```python
from build123d import *

# Parameters (mm, degrees)
SKETCH1_W           = 30
SKETCH1_H           = 100
BOSS_EXTRUDE1_DEPTH = 3.75
BOSS_EXTRUDE2_START = -3
SKETCH2_W           = 15
SKETCH2_H           = 50
BOSS_EXTRUDE2_DEPTH = 4


with BuildPart() as part:
    # Sketch1 → Boss-Extrude1 (new, symmetric)
    with BuildSketch(Plane(origin=(0, 0, 0), x_dir=(1, 0, 0), z_dir=(0, 1, 0))):
        with Locations((-15, 0)):
            Rectangle(SKETCH1_W, SKETCH1_H)
    extrude(amount=BOSS_EXTRUDE1_DEPTH, both=True)

    # Sketch2 → Boss-Extrude2 (add)
    with BuildSketch(Plane(origin=(0, 3.75, 0), x_dir=(1, 0, 0), z_dir=(0, 1, 0)).offset(BOSS_EXTRUDE2_START)):
        with Locations((7.5, 0)):
            Rectangle(SKETCH2_W, SKETCH2_H)
    extrude(amount=-BOSS_EXTRUDE2_DEPTH)


solid = part.part
```
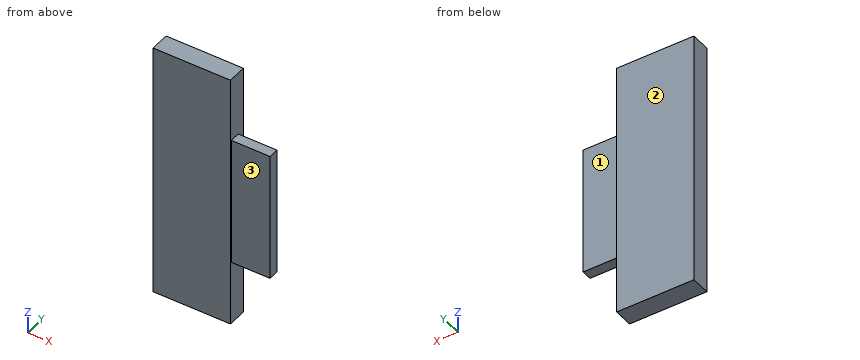
Source: CAD feature listing. Evaluate the final solid. Frame: model axes, mm. Face numbers are marked on the shaded views. A direction names the side the tool comes from. Coordinates: 2 decimals unless noted, no trailing zeros. Loops run counter-clockwise (first coordinate to the right, second up) from the corner with the lowest first, then second, coordinate; pieces in that order, holes last. Notation, with made-up numbers: M -20,17.25 L 39,17.25 A19 ccw 39,26.25 Z; hole C 57,36 d10. An arc over 180 degrees is marked long. Use CSV: the item, a comma, the result in double quotes.
(1) Cut plane C-C on x = 9. Return loops of the section in (y, z), and give its area (3 significant figures).
Answers follow:
outline,"M -3.25,-25 L 0.75,-25 L 0.75,25 L -3.25,25 Z"
area,"200 mm²"
(2) Cut plane D-D on z = 44. Return loops of the section in (x, y), and give its area (3 significant figures).
Answers follow:
outline,"M -30,-3.75 L 0,-3.75 L 0,3.75 L -30,3.75 Z"
area,"225 mm²"
(3) Line query: line 1 (X direction, y = 3, z = 31); line 2 (Z direction, x = 5, y = -0.25). Output: solid intervals per line, ascending. Write a range as [from, to].
Answers follow:
line 1,"[-30, 0]"
line 2,"[-25, 25]"
(4) Reachability of the marked faces 1, 2 and 3 from +Z, -Z, +X, -X, +Y, -Y: full face, straight path, thin tool, end or side. Return the list, or none.
Answers follow:
face 1,"+Z, -Z, +X, +Y"
face 2,"+Z, -Z, +X, -X, +Y"
face 3,"+Z, -Z, +X, -Y"
(5) Contact query for flat-ended pins moving along their axis: pin 1 (3 mm diameter, centred on x = 5.5, y = -1.5, fed in from -Z); pin 2 (3 mm diameter, centred on x = 0.5, z = -35.5, fed in from -Y); pin 3 (7.5 mm diameter, centred on x = 6.5, z = 6, fed in from +Y); pin 4 (1.2 mm diameter, centred on x = 10, y = -0.5, fed in from +Z). Output: stop coordinate, or through.
Answers follow:
pin 1,"z = -25"
pin 2,"y = -3.75"
pin 3,"y = 0.75"
pin 4,"z = 25"
(6) Cut plane B-B on z = -24. Return loops of the section in (x, y), and give its area (3 significant figures).
Answers follow:
outline,"M -30,-3.75 L 0,-3.75 L 0,-3.25 L 15,-3.25 L 15,0.75 L 0,0.75 L 0,3.75 L -30,3.75 Z"
area,"285 mm²"
(7) Cut plane A-A on y = -0.5. Return loops of the section in (x, z).
Answers follow:
outline,"M -30,-50 L 0,-50 L 0,-25 L 15,-25 L 15,25 L 0,25 L 0,50 L -30,50 Z"
